Can you work these out from the model? Positions are in its coordinate system, mm. A direction names the side the tool comes from. Give positions to 0.01 mm unless a question says otherwise; leave off trailing zeros. Order: outer loops, then holes, each group sorted by start corner. A loop starts at its lowest first (then second) coordinate and runs counter-clockwise, first axis right, second up. Notation, with made-up numbers: M 29,80.5 L 38,80.5 A22 ccw 38,102.5 Z; hole C 35.25,-31 d9. An arc over 180 degrees is marked long. Answer as a JSON object with one key per item and string values.
```python
from build123d import *

# Parameters (mm, degrees)
F0_W     = 34.2265013605
F0_H     = 44.7577312589
F1_DEPTH = 25
F2_SIZE  = 30
F3_SIZE  = 30
F4_R     = 9.0461228016
F5_DEPTH = 34.2275013605
F6_R     = 10.2345227576
F7_DEPTH = 84.2827808433


with BuildPart() as f1:
    # F0 (on Front) → F1 (new body, symmetric)
    with BuildSketch(Plane.XZ):
        with Locations((-32.9100964591, 46.9517372549)):
            Rectangle(F0_W, F0_H)
        with BuildLine():
            Line((-15.7968457788, 24.5728716254), (-50.0233471394, 24.5728716254))
            Line((-50.0233471394, 24.5728716254), (-50.0233471394, -24.5728716254))
            Line((-50.0233471394, -24.5728716254), (-27.4733056784, -24.5728716254))
            ThreePointArc((-27.4733056784, -24.5728716254), (0, 2.900434053), (27.4733056784, -24.5728716254))
            Line((27.4733056784, -24.5728716254), (50.0233471394, -24.5728716254))
            Line((50.0233471394, -24.5728716254), (50.0233471394, 24.5728716254))
            Line((50.0233471394, 24.5728716254), (-15.7968457788, 24.5728716254))
        make_face()
    extrude(amount=F1_DEPTH, both=True)

    # F2
    f2_edges = [f1.edges().sort_by_distance(p)[0] for p in [
        (-32.910096, -25, 69.330603),
    ]]
    chamfer(f2_edges, length=F2_SIZE)

    # F3
    f3_edges = [f1.edges().sort_by_distance(p)[0] for p in [
        (50.023347, 0, 24.572872),
    ]]
    chamfer(f3_edges, length=F3_SIZE)

    # F4 (on face) → F5 (cut, through all)
    with BuildSketch(Plane.YZ.offset(-15.7968457788)):
        with Locations((0, 46.9517372549)):
            Circle(F4_R)
    extrude(amount=-F5_DEPTH, mode=Mode.SUBTRACT)

    # F6 (on face) → F7 (cut, through all)
    with BuildSketch(Plane(origin=(22.2981093824, 0, 22.2981093824), x_dir=(0, 1, 0), z_dir=(0.7071067812, 0, 0.7071067812))):
        with Locations((0, -17.9962038203)):
            Circle(F6_R)
    extrude(amount=-F7_DEPTH, mode=Mode.SUBTRACT)


solid = f1.part
```
1) For faces 1 (the face through (-15.797, 5, 37)), 2 (the face through (-32.67, -1.18, 55.92)), which set-ups out of +Z, -Z, +X, -X, +Y, -Y let a thin tool reach every point of the face, with its end or its side?
Results found:
{"face 1": "+Z, +X, +Y, -Y", "face 2": "+X, -X"}
2) I'm going to push flat-ended pins straight in: pin 1 Ø10 at (x, y) = (-1.5, 18) entering from -Z; pin 2 Ø23.5 at (y, z) = (0, 46.95) entering from +X; pin 3 Ø12 at (x, z) = (29, 18) entering from +Y; pin 4 Ø1.5 at (x, y) = (23, -20) entering from -Z. Where does each tip first touch, or does it pass through?
Results found:
{"pin 1": "stops at z = 2.12", "pin 2": "stops at x = -15.8", "pin 3": "stops at y = 25", "pin 4": "stops at z = -10.76"}
3) I want a section at D-D on x = -35. Write out the boundary of the cut face in (y, z), and give its area (3 significant figures).
Results found:
{"outline": "M -25,-24.57 L 25,-24.57 L 25,69.33 L 5,69.33 L -25,39.33 Z; hole C 0,46.95 d18.09", "area": "3,990 mm²"}
4) I want a section at C-C on y = 0. Write out the boundary of the cut face in (x, z).
Results found:
{"outline": "M -50.02,-24.57 L -27.47,-24.57 A27.47 cw 11.4,0.42 L 27.79,16.81 L 20.02,24.57 L -15.8,24.57 L -15.8,37.91 L -50.02,37.91 Z; M -50.02,56 L -15.8,56 L -15.8,64.33 L -50.02,64.33 Z; M 25.52,-14.4 A27.47 cw 27.47,-24.57 L 50.02,-24.57 L 50.02,-5.43 L 42.26,2.34 Z"}
5) I need wall thicknesses on L1, parallel to X at y = 4, z = 33.5; L2, parallel to Y at x = -28, z = 40; L3, parallel to Z at x = -30.5, y = 0. Which ranges of each line are inside material? Lowest first, please.
Results found:
{"L1": "x = -50.02 to -15.8", "L2": "y = -24.33 to -5.79, 5.79 to 25", "L3": "z = -24.57 to 37.91, 56 to 64.33"}
6) Thinking about a two-plate mould opening in Z: for faces 3 (the face through (-50.023, 0, 13)), 4 (the face through (-0.604, -0.35, 2.894)), 5 (the face through (33.84, -2.22, -5.74)), 6 (the face through (-33.15, -10.21, 54.12)), which applies, pulls with the +Z half, pulls with the -Z half, needs draft (parallel to the pull), parting line crosses it, or undercut?
Results found:
{"face 3": "needs draft", "face 4": "pulls with the -Z half", "face 5": "undercut", "face 6": "pulls with the +Z half"}
7) I want a section at A-A on z = 51.5. Write out the boundary of the cut face in (x, y), and give its area (3 significant figures).
Results found:
{"outline": "M -50.02,-12.83 L -15.8,-12.83 L -15.8,-7.82 L -50.02,-7.82 Z; M -50.02,7.82 L -15.8,7.82 L -15.8,25 L -50.02,25 Z", "area": "760 mm²"}
8) I want a section at B-B on y = 17. Write out the boundary of the cut face in (x, z).
Results found:
{"outline": "M -50.02,-24.57 L -27.47,-24.57 A27.47 cw 27.47,-24.57 L 50.02,-24.57 L 50.02,-5.43 L 20.02,24.57 L -15.8,24.57 L -15.8,69.33 L -50.02,69.33 Z"}
